For this review, take the finished solid that the model builds, in its own axes (mm). A direction names the side the tool comes from. Round coordinates to 2 decimals unless told otherwise and drop trailing zeros. Write each loop counter-clockwise with the first axis right and the second up, starting at its lowest first coordinate (ties: lowest second). Pieces come first, ordered by that corner, then holes. Notation, with made-up numbers: (11, 24.25) -> (26, 24.25) arc R24 cw to (26, 52.25) -> close; hole circle Ø2 at (31, -16.75). An arc over 180 degrees is marked (long way). Answer in a Markdown table with one row per item. Add a question column.
```python
from build123d import *

# Parameters (mm, degrees)
SKETCH_1_R         = 6
EXTRUDE_2_DEPTH    = 80
DOME_1_FACE_RADIUS = 4.603594806
DOME_1_HEIGHT      = 5


# Read off the part's stored shape, not the designer's step: 拔模2
with BuildPart() as part:
    # 草图1 → 凸台-拉伸2 (new, symmetric)
    with BuildSketch(Plane.XY):
        Circle(SKETCH_1_R)
    extrude(amount=EXTRUDE_2_DEPTH, both=True)

    # 拔模2 outline → 拔模2 (revolve, cut)
    with BuildSketch(Plane.XZ):
        Polygon((6, 80), (4.603594806, 80), (6, 0), align=None)
    revolve(axis=Axis((0, 0, 0), (0, 0, 1)), mode=Mode.SUBTRACT)

    # 圆顶1: a dome of height H over a round flat face of radius A is a cap of a sphere of radius (A * A + H * H) / (2 * H)
    dome_1_r = (DOME_1_FACE_RADIUS * DOME_1_FACE_RADIUS + DOME_1_HEIGHT * DOME_1_HEIGHT) / (2 * DOME_1_HEIGHT)
    dome_1_base = Plane((0, 0, 80), z_dir=(0, 0, 1))
    with Locations(dome_1_base.offset(DOME_1_HEIGHT - dome_1_r)):
        dome_1_ball = Sphere(dome_1_r, mode=Mode.PRIVATE)
    add(split(dome_1_ball, bisect_by=dome_1_base, keep=Keep.TOP, mode=Mode.PRIVATE))


solid = part.part
```
1. Clearance check with flat-ended pins moving along their axes: pin 1 Ø6 at (x, y) = (-4, -4.5) entering from +Z; pin 2 Ø3 at (y, z) = (-3, -38) entering from -X; pin 3 Ø6 at (y, z) = (-4.5, 24.5) entering from -X. State where each tip first meets the part, or that it passes through.
2. For L1, parallel to Y at x = -0.5, z = -40.5; L2, parallel to Z at x = 1, y = 0; L3, parallel to Y at x = 3.75, z = -47, list the stretches that pass through material, from the lowest coordinate up. Write a range as [from, to].
3. Tool access review of faces 1 (the flat face through (0, 0, -80)), 2 (the conical face through (-4.215, -3.232, 39.44)): name each direction out of +Z, -Z, +X, -X, +Y, -Y from which nothing blocks a thin tool from reaching the whole face with its end or side.
4. We need section A-A (z = -15). Write out the cut boundary in (x, y).
5. We need section B-B (z = 73.5). Write out the cut boundary in (x, y).
Response:
| question | item | result |
|---|---|---|
| 1 | pin 1 | z = 83.88 |
| 1 | pin 2 | x = -5.81 |
| 1 | pin 3 | x = -5.37 |
| 2 | L1 | [-5.98, 5.98] |
| 2 | L2 | [-80, 84.89] |
| 2 | L3 | [-4.68, 4.68] |
| 3 | face 1 | -Z, +X, -X, +Y, -Y |
| 3 | face 2 | +Z |
| 4 | outline | circle Ø12 at (0, 0) |
| 5 | outline | circle Ø9.43 at (0, 0) |
